Geometry: final body of the model. Coordinates: model frame, mm. A direction names the side the tool comes from. Round coordinates to 2 decimals unless told otherwise and drop trailing zeros. Loops run counter-clockwise (first coordinate to the right, second up) from the corner with the lowest first, then second, coordinate; pieces in that order, holes last. Notation, with made-up numbers: M -16,13.5 L 31,13.5 A22 ccw 31,51.5 Z; hole C 16,4.5 d5. An arc over 180 degrees is marked long. Write each question's results on one line, items separated by ' | '.
```python
from build123d import *

# Parameters (mm, degrees)
SKETCH_1_W                      = 106
SKETCH_1_H                      = 105
EXTRUDE_1_DEPTH                 = 40
CUT_EXTRUDE_1_DEPTH             = 125.233650836
CUT_EXTRUDE_1_DEPTH_BACK        = 125.233650836
SKETCH_3_W                      = 100
SKETCH_3_H                      = 99
CUT_EXTRUDE_3_DEPTH             = 1
CUT_EXTRUDE_3_DEPTH_BACK        = 3
SKETCH_7_R                      = 2.5
SKETCH_7_R_2                    = 1.6
CUT_EXTRUDE_4_REACH             = 126.234
SKETCH_6_W                      = 13
SKETCH_6_H                      = 24
CUT_EXTRUDE_4_DIRECTION_2_DEPTH = 125.233650836
CUT_EXTRUDE_5_DEPTH             = 155.470061824
CUT_EXTRUDE_5_DEPTH_BACK        = 155.470061824
SKETCH_10_W                     = 13
SKETCH_10_H                     = 24
CUT_EXTRUDE_6_REACH             = 156.47
CUT_EXTRUDE_6_DIRECTION_2_DEPTH = 155.470061824


with BuildPart() as part:
    # 草图1 → 凸台-拉伸1 (new body)
    with BuildSketch(Plane.XY):
        with Locations((0, 52.5)):
            Rectangle(SKETCH_1_W, SKETCH_1_H)
    extrude(amount=EXTRUDE_1_DEPTH)

    # 草图3 → 切除-拉伸1 (cut, two sides: drawn at the far end of the back side and taken through both)
    with BuildSketch(Plane(origin=(0, 0, 0), x_dir=(-1, 0, 0), z_dir=(0, 0, -1)).offset(-CUT_EXTRUDE_1_DEPTH_BACK)):
        with Locations((0, 52.5)):
            Rectangle(SKETCH_3_W, SKETCH_3_H)
    extrude(amount=CUT_EXTRUDE_1_DEPTH + CUT_EXTRUDE_1_DEPTH_BACK, mode=Mode.SUBTRACT)

    # 草图7 → 切除-拉伸3 (cut, two sides: drawn at the far end of the back side and taken through both)
    with BuildSketch(Plane.XZ.offset(-CUT_EXTRUDE_3_DEPTH_BACK)):
        with Locations(Location((0, 20, 0), (0, 0, 180))):
            Circle(SKETCH_7_R)
        with Locations(Location((5, 25, 0), (0, 0, 180))):
            Circle(SKETCH_7_R_2)
        with Locations(Location((5, 15, 0), (0, 0, 180))):
            Circle(SKETCH_7_R_2)
        with Locations(Location((-5, 15, 0), (0, 0, 180))):
            Circle(SKETCH_7_R_2)
        with Locations(Location((-5, 25, 0), (0, 0, 180))):
            Circle(SKETCH_7_R_2)
        with Locations(Location((15, 25, 0), (0, 0, 180))):
            Circle(SKETCH_7_R_2)
        with Locations(Location((-15, 25, 0), (0, 0, 180))):
            Circle(SKETCH_7_R_2)
        with Locations(Location((15, 15, 0), (0, 0, 180))):
            Circle(SKETCH_7_R_2)
        with Locations(Location((-15, 15, 0), (0, 0, 180))):
            Circle(SKETCH_7_R_2)
    extrude(amount=CUT_EXTRUDE_3_DEPTH + CUT_EXTRUDE_3_DEPTH_BACK, mode=Mode.SUBTRACT)

    # 草图6 → 切除-拉伸4 (cut, up to next)
    with BuildSketch(Plane(origin=(0, 105, 0), x_dir=(1, 0, 0), z_dir=(0, 1, 0)), mode=Mode.PRIVATE) as cut_extrude_4_sk1:
        with Locations((0, -20)):
            Rectangle(SKETCH_6_W, SKETCH_6_H)
    cut_extrude_4_tool1 = extrude(cut_extrude_4_sk1.sketch, amount=-CUT_EXTRUDE_4_REACH, mode=Mode.PRIVATE) & part.part
    add(cut_extrude_4_tool1.solids().sort_by_distance((0, 105, 20))[0], mode=Mode.SUBTRACT)

    # 草图6 → 切除-拉伸4 direction 2 (cut)
    with BuildSketch(Plane(origin=(0, 105, 0), x_dir=(1, 0, 0), z_dir=(0, 1, 0))):
        with Locations((0, -20)):
            Rectangle(SKETCH_6_W, SKETCH_6_H)
    extrude(amount=CUT_EXTRUDE_4_DIRECTION_2_DEPTH, mode=Mode.SUBTRACT)

    # 草图10 → 切除-拉伸5 (cut, two sides: drawn at the far end of the back side and taken through both)
    with BuildSketch(Plane.ZY.offset(53).offset(-CUT_EXTRUDE_5_DEPTH_BACK)):
        with Locations((20, 87.806952357)):
            Rectangle(SKETCH_10_W, SKETCH_10_H)
    extrude(amount=CUT_EXTRUDE_5_DEPTH + CUT_EXTRUDE_5_DEPTH_BACK, mode=Mode.SUBTRACT)

    # 草图12 → 切除-拉伸6 (cut, up to next)
    with BuildSketch(Plane(origin=(53, 0, 0), x_dir=(0, 0, -1), z_dir=(1, 0, 0)), mode=Mode.PRIVATE) as cut_extrude_6_sk1:
        with BuildLine():
            Line((-27.5, 25.649961527), (-27.5, 47.398469004))
            ThreePointArc((-27.5, 47.398469004), (-20, 54.898469004), (-12.5, 47.398469004))
            Line((-12.5, 47.398469004), (-12.5, 25.649961527))
            ThreePointArc((-12.5, 25.649961527), (-20, 18.149961527), (-27.5, 25.649961527))
        make_face()
    cut_extrude_6_tool1 = extrude(cut_extrude_6_sk1.sketch, amount=-CUT_EXTRUDE_6_REACH, mode=Mode.PRIVATE) & part.part
    add(cut_extrude_6_tool1.solids().sort_by_distance((53, 36.524215, 20))[0], mode=Mode.SUBTRACT)

    # 草图12 → 切除-拉伸6 direction 2 (cut)
    with BuildSketch(Plane(origin=(53, 0, 0), x_dir=(0, 0, -1), z_dir=(1, 0, 0))):
        with BuildLine():
            Line((-27.5, 25.649961527), (-27.5, 47.398469004))
            ThreePointArc((-27.5, 47.398469004), (-20, 54.898469004), (-12.5, 47.398469004))
            Line((-12.5, 47.398469004), (-12.5, 25.649961527))
            ThreePointArc((-12.5, 25.649961527), (-20, 18.149961527), (-27.5, 25.649961527))
        make_face()
    extrude(amount=CUT_EXTRUDE_6_DIRECTION_2_DEPTH, mode=Mode.SUBTRACT)


solid = part.part
```
1. Section A-A (y = 7). Output: boundary loops of the cut face in (x, z), then the cut area to 3 significant figures.
Answer key:
outline: M -53,0 L -50,0 L -50,40 L -53,40 Z; M 50,0 L 53,0 L 53,40 L 50,40 Z | area: 240 mm²
2. Access query for faces 5 (the face through (-13.4, 1.52, 14.93)), 6 (the face through (0, 104, 32)), 7 (the face through (51.52, 18.15, 19.84)), 8 (the face through (11, 105, 20)), 9 (the face through (-51, 75.807, 20)). Directions: +Z, -Z, +X, -X, +Y, -Y. A direction counts if a zero-diameter tool reaches every point of the face in a straight line with its end or side. Return the directions, or none.
Answer key:
face 5: -Y | face 6: +Y | face 7: +X | face 8: +Z, -Z, +X, -X, +Y | face 9: +X, -X
3. Section D-D (x = 28). Output: boundary loops of the cut face in (y, z), then the cut area to 3 significant figures.
Answer key:
outline: M 0,0 L 3,0 L 3,40 L 0,40 Z; M 102,0 L 105,0 L 105,40 L 102,40 Z | area: 240 mm²
4. Section B-B (z = 20). Output: boundary loops of the cut face in (x, y), then the cut area to 3 significant figures.
Answer key:
outline: M -53,0 L -2.5,0 L -2.5,3 L -50,3 L -50,75.81 L -53,75.81 Z; M -53,99.81 L -50,99.81 L -50,102 L -6.5,102 L -6.5,105 L -53,105 Z; M 2.5,0 L 53,0 L 53,18.15 L 50,18.15 L 50,3 L 2.5,3 Z; M 6.5,102 L 50,102 L 50,99.81 L 53,99.81 L 53,105 L 6.5,105 Z; M 50,54.9 L 53,54.9 L 53,75.81 L 50,75.81 Z | area: 922 mm²
5. Draft query along Z for faces 1 (the face through (16.18, 1.52, 13.92)), 2 (the face through (-4, 2, 40)), 3 (the face through (-1, 0, 24)), 4 (the face through (16.18, 1.52, 23.92)). Return one class per face: pulls with the +Z half, pulls with the -Z half, needs draft (parallel to the pull), parting line crosses it, or undercut.
Answer key:
face 1: undercut | face 2: pulls with the +Z half | face 3: needs draft | face 4: undercut
6. Section C-C (x = -5). Output: boundary loops of the cut face in (y, z), then the cut area to 3 significant figures.
Answer key:
outline: M 0,0 L 3,0 L 3,13.4 L 0,13.4 Z; M 0,16.6 L 3,16.6 L 3,23.4 L 0,23.4 Z; M 0,26.6 L 3,26.6 L 3,40 L 0,40 Z; M 102,0 L 105,0 L 105,8 L 102,8 Z; M 102,32 L 105,32 L 105,40 L 102,40 Z | area: 149 mm²
7. Ray query, probe 1 along Z at (x, y) = (-15, 1.1); probe 2 along X at (y, z) = (0.95, 15); probe 3 along X at (y, z) = (14, 37). Return the intervals inside material, ascending.
Answer key:
probe 1: z = 0 to 13.4, 16.6 to 23.4, 26.6 to 40 | probe 2: x = -53 to -16.6, -13.4 to -6.6, -3.4 to 3.4, 6.6 to 13.4, 16.6 to 53 | probe 3: x = -53 to -50, 50 to 53
